Source: CAD feature listing. Evaluate the final solid. Frame: model axes, mm. Face numbers are marked on the shaded views. A direction names the side the tool comes from. Give positions to 0.01 mm unless a question says otherwise; leave off trailing zeros. Loops run counter-clockwise (first coordinate to the right, second up) from the corner with the lowest first, then second, coordinate; pieces in that order, holes last.
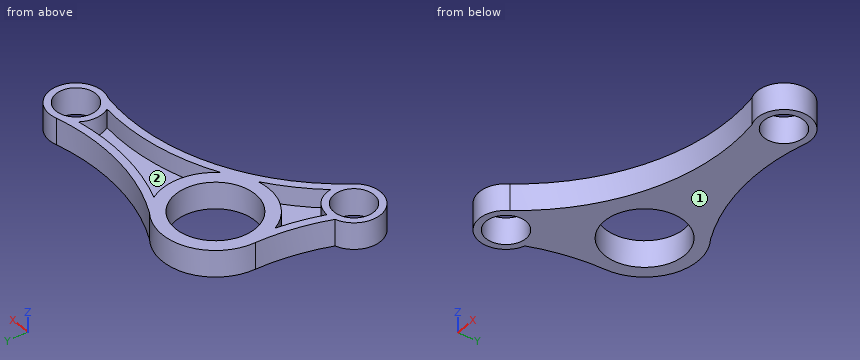
from build123d import *

# Parameters (mm, degrees)
SKETCH3_R           = 20
SKETCH3_R_2         = 15
SKETCH3_R_3         = 10
SKETCH3_R_4         = 7.5
BOSS_EXTRUDE1_DEPTH = 10
BOSS_EXTRUDE3_DEPTH = 3


with BuildPart() as part:
    # Sketch3 → Boss-Extrude1 (new body)
    # profile 1 of 6: a face of its own
    with BuildSketch(Plane.XY):
        with BuildLine():
            ThreePointArc((93.599540264, 15.920778558), (128.582431805, 43.32581827), (172.792265807, 47.834640706))
            ThreePointArc((172.792265807, 47.834640706), (170.402615718, 49.368900415), (168.540603284, 51.513029633))
            ThreePointArc((168.540603284, 51.513029633), (144.624934442, 50.959037098), (121.8606014, 43.607080548))
            ThreePointArc((121.8606014, 43.607080548), (117.069520627, 39.683138814), (111.307748037, 37.412951524))
            ThreePointArc((111.307748037, 37.412951524), (102.56627164, 30.460503982), (94.837400467, 22.39734785))
            ThreePointArc((94.837400467, 22.39734785), (94.918388119, 21.666366387), (94.945432764, 20.931409595))
            ThreePointArc((94.945432764, 20.931409595), (94.603100055, 18.337288838), (93.599540264, 15.920778558))
        make_face()
    # profile 2 of 6: a face of its own
    with BuildSketch(Plane.XY):
        with BuildLine():
            ThreePointArc((89.245155024, 47.620117101), (87.528873404, 52.135867645), (86.945432764, 56.931409595))
            ThreePointArc((86.945432764, 56.931409595), (85.538303333, 43.476636452), (81.884211959, 30.451332241))
            ThreePointArc((81.884211959, 30.451332241), (83.546001392, 30.833005014), (85.248475349, 30.9268168))
            ThreePointArc((85.248475349, 30.9268168), (87.679513668, 39.169871065), (89.245155024, 47.620117101))
        make_face()
    # profile 3 of 6: a face of its own
    with BuildSketch(Plane.XY):
        with BuildLine():
            ThreePointArc((168.529854034, 62.33307921), (170.898087492, 64.895680758), (174.002612838, 66.488595942))
            ThreePointArc((174.002612838, 66.488595942), (145.688050003, 64.85214344), (118.581891775, 73.197719001))
            ThreePointArc((118.581891775, 73.197719001), (121.570888747, 70.573111736), (123.981351449, 67.408884223))
            ThreePointArc((123.981351449, 67.408884223), (145.906367795, 61.805873057), (168.529854034, 62.33307921))
        make_face()
    # profile 4 of 6: a face of its own
    with BuildSketch(Plane.XY):
        with Locations((106.945432764, 56.931409595)):
            Circle(SKETCH3_R)
        with Locations((106.945432764, 56.931409595)):
            Circle(SKETCH3_R_2, mode=Mode.SUBTRACT)
    # profile 5 of 6: a face of its own
    with BuildSketch(Plane.XY):
        with Locations((84.945432764, 20.931409595)):
            Circle(SKETCH3_R_3)
        with Locations((84.945432764, 20.931409595)):
            Circle(SKETCH3_R_4, mode=Mode.SUBTRACT)
    # profile 6 of 6: a face of its own
    with BuildSketch(Plane.XY):
        with Locations((176.945432764, 56.931409595)):
            Circle(SKETCH3_R_3)
        with Locations((176.945432764, 56.931409595)):
            Circle(SKETCH3_R_4, mode=Mode.SUBTRACT)
    extrude(amount=BOSS_EXTRUDE1_DEPTH)

    # Sketch4 → Boss-Extrude3 (add)
    with BuildSketch(Plane.XY):
        with BuildLine():
            ThreePointArc((94.837400467, 22.39734785), (91.59167372, 28.403188577), (85.248475349, 30.9268168))
            ThreePointArc((85.248475349, 30.9268168), (87.679513668, 39.169871065), (89.245155024, 47.620117101))
            ThreePointArc((89.245155024, 47.620117101), (98.547702834, 38.779877097), (111.307748037, 37.412951524))
            ThreePointArc((111.307748037, 37.412951524), (102.56627164, 30.460503982), (94.837400467, 22.39734785))
        make_face()
        with BuildLine():
            ThreePointArc((168.529854034, 62.33307921), (166.945437699, 56.921475033), (168.540603284, 51.513029633))
            ThreePointArc((168.540603284, 51.513029633), (144.624934442, 50.959037098), (121.8606014, 43.607080548))
            ThreePointArc((121.8606014, 43.607080548), (126.866513553, 55.156433479), (123.981351449, 67.408884223))
            ThreePointArc((123.981351449, 67.408884223), (145.906367795, 61.805873057), (168.529854034, 62.33307921))
        make_face()
    extrude(amount=BOSS_EXTRUDE3_DEPTH)


solid = part.part
1) Cut plane B-B (y = 26). Return loops of the section in (x, z) (3 decimals).
Checks:
outline: (76.325, 0) - (79.417, 0) - (79.417, 10) - (76.325, 10) - close; (90.473, 0) - (102.225, 0) - (102.225, 10) - (98.035, 10) - (98.035, 3) - (93.566, 3) - (93.566, 10) - (90.473, 10) - close
2) Ray query, probe 1 along Y at (x, z) = (104, 8.25); probe 2 along X at (y, z) = (43, 8.75); probe 3 along Y at (x, z) = (182, 3.5). Return the intervals inside material, ascending.
Checks:
probe 1: y = 27.7 to 31.74, 37.15 to 42.22, 71.64 to 76.71
probe 2: x = 85.45 to 88.5, 92.6 to 101.39, 112.51 to 127.79
probe 3: y = 48.3 to 51.39, 62.47 to 65.56
3) Cut plane A-A (x = 101). Return loops of the section in (y, z).
Checks:
outline: (24.76, 0) - (43.16, 0) - (43.16, 10) - (37.84, 10) - (37.84, 3) - (29, 3) - (29, 10) - (24.76, 10) - close; (70.7, 0) - (76.03, 0) - (76.03, 10) - (70.7, 10) - close
4) Reachability of the marked faces 1 and 2 from +Z, -Z, +X, -X, +Y, -Y: full face, straight path, thin tool, end or side. Return the list, or none.
Checks:
face 1: -Z, +X, -X, +Y, -Y
face 2: +Z
5) Cut plane D-D (x = 154.5). Return loops of the section in (y, z).
Checks:
outline: (49.03, 0) - (64.28, 0) - (64.28, 10) - (61.28, 10) - (61.28, 3) - (52.03, 3) - (52.03, 10) - (49.03, 10) - close
6) Contact query for flat-ended pins moving along their axis: P1, Ø5, axis at y = 31.5, z = 2, coming from the +X side (3 decimals); P2, Ø2, axis at x = 130, z = 4.5, coming from the +Y side; P3, Ø2, axis at y = 66, z = 2.5, coming from the -X side; P4, Ø12, axis at x = 176.95, y = 56.93, coming from the +Z side. Output: stop coordinate, or through.
Checks:
P1: stops at x = 111.675
P2: stops at y = 68.72
P3: stops at x = 88.65
P4: passes through
7) Cut plane C-C (z = 6.25). Return loops of the section in (x, y), and give its area (3 significant figures).
Checks:
outline: (81.88, 30.45) arc R10 ccw (long way) to (93.6, 15.92) arc R80 cw to (172.79, 47.83) arc R10 ccw (long way) to (174, 66.49) arc R80 cw to (118.58, 73.2) arc R20 ccw to (86.95, 56.93) arc R80 cw to start; hole circle Ø15 at (84.95, 20.93); hole (85.25, 30.93) arc R10 cw to (94.84, 22.4) arc R83 cw to (111.31, 37.41) arc R20 cw to (89.25, 47.62) arc R83 cw to start; hole circle Ø30 at (106.95, 56.93); hole (121.86, 43.61) arc R83 cw to (168.54, 51.51) arc R10 cw to (168.53, 62.33) arc R83 cw to (123.98, 67.41) arc R20 cw to start; hole circle Ø15 at (176.95, 56.93)
area: 1,280 mm2
